from build123d import *

# Parameters (mm, degrees)
F0_W     = 38.4
F0_H     = 28.4
F0_R     = 1.1
F0_R_2   = 4.1
F1_DEPTH = 1.5
F2_W     = 38.4
F2_H     = 1.5
F3_DEPTH = 11
F6_W     = 38.4
F6_H     = 14.2
F7_DEPTH = 25.001
F8_R     = 4.1
F8_R_2   = 1.1
F9_DEPTH = 1.5
F10_R    = 1


with BuildPart() as f1:
    # F0 (on Top) → F1 (new body)
    with BuildSketch(Plane.XY):
        Rectangle(F0_W, F0_H)
        with Locations((-16.2, -7.2)):
            Circle(F0_R, mode=Mode.SUBTRACT)
        with Locations((14.9, -7.2)):
            Circle(F0_R, mode=Mode.SUBTRACT)
        with Locations((-10, 0)):
            Circle(F0_R_2, mode=Mode.SUBTRACT)
        with Locations((-16.2, 7.2)):
            Circle(F0_R, mode=Mode.SUBTRACT)
        with BuildLine():
            ThreePointArc((-3, 4.8), (-1.5355339059, 8.3355339059), (2, 9.8))
            Line((2, 9.8), (11.7, 9.8))
            ThreePointArc((11.7, 9.8), (12.4071067812, 9.5071067812), (12.7, 8.8))
            Line((12.7, 8.8), (12.7, 5.5901699437))
            ThreePointArc((12.7, 5.5901699437), (12.7871290708, 5.1819216533), (13.0333333333, 4.8448139512))
            ThreePointArc((13.0333333333, 4.8448139512), (15.2, 0), (13.0333333333, -4.8448139512))
            ThreePointArc((13.0333333333, -4.8448139512), (12.7871290708, -5.1819216533), (12.7, -5.5901699437))
            Line((12.7, -5.5901699437), (12.7, -8.8))
            ThreePointArc((12.7, -8.8), (12.4071067812, -9.5071067812), (11.7, -9.8))
            Line((11.7, -9.8), (2, -9.8))
            ThreePointArc((2, -9.8), (-1.5355339059, -8.3355339059), (-3, -4.8))
            Line((-3, -4.8), (-3, 4.8))
        make_face(mode=Mode.SUBTRACT)
        with Locations((14.9, 7.2)):
            Circle(F0_R, mode=Mode.SUBTRACT)
    extrude(amount=F1_DEPTH)

    # F2 (on face) → F3 (join)
    with BuildSketch(Plane(origin=(0, 0, 0), x_dir=(1, 0, 0), z_dir=(0, 0, -1))):
        with Locations((0, 13.45)):
            Rectangle(F2_W, F2_H)
    extrude(amount=F3_DEPTH)

    # F5: F1 across plane


with BuildPart() as f1_1:
    add(f1.part)
    add(f1.part.mirror(Plane.XY.offset(-11)))

    # F6 (on face) → F7 (cut, through all)
    with BuildSketch(Plane(origin=(0, 0, -23.5), x_dir=(1, 0, 0), z_dir=(0, 0, -1))):
        with Locations((0, -7.1)):
            Rectangle(F6_W, F6_H)
    extrude(amount=-F7_DEPTH, mode=Mode.SUBTRACT)

    # F8 (on face) → F9 (cut, through all)
    with BuildSketch(Plane.XZ.offset(14.2)):
        with Locations((-10, -11)):
            Circle(F8_R)
        with Locations((-16.2, -3.8)):
            Circle(F8_R_2)
        with Locations((15.4, -3.8)):
            Circle(F8_R_2)
        with BuildLine():
            Line((12.2, -1.2), (2.5, -1.2))
            ThreePointArc((2.5, -1.2), (-1.0355339059, -2.6644660941), (-2.5, -6.2))
            Line((-2.5, -6.2), (-2.5, -15.8))
            ThreePointArc((-2.5, -15.8), (-1.0355339059, -19.3355339059), (2.5, -20.8))
            Line((2.5, -20.8), (12.2, -20.8))
            ThreePointArc((12.2, -20.8), (12.9071067812, -20.5071067812), (13.2, -19.8))
            Line((13.2, -19.8), (13.2, -16.5901699437))
            ThreePointArc((13.2, -16.5901699437), (13.2871290708, -16.1819216533), (13.5333333333, -15.8448139512))
            ThreePointArc((13.5333333333, -15.8448139512), (15.7, -11), (13.5333333333, -6.1551860488))
            ThreePointArc((13.5333333333, -6.1551860488), (13.2871290708, -5.8180783467), (13.2, -5.4098300563))
            Line((13.2, -5.4098300563), (13.2, -2.2))
            ThreePointArc((13.2, -2.2), (12.9071067812, -1.4928932188), (12.2, -1.2))
        make_face()
        with Locations((-16.2, -18.2)):
            Circle(F8_R_2)
        with Locations((15.4, -18.2)):
            Circle(F8_R_2)
    extrude(amount=-F9_DEPTH, mode=Mode.SUBTRACT)

    # F10
    f10_edges = [f1_1.edges().sort_by_distance(p)[0] for p in [
        (-19.2, 0, -22.75),
        (-19.2, 0, 0.75),
        (-5.9, 0, 0.75),
        (-14.1, 0, 0.75),
        (-5.9, 0, -22.75),
        (-14.1, 0, -22.75),
        (-3, 0, -22.75),
        (15.2, 0, -22.75),
        (15.2, 0, 0.75),
        (19.2, 0, -22.75),
        (19.2, 0, 0.75),
        (-3, 0, 0.75),
    ]]
    fillet(f10_edges, radius=F10_R)


solid = f1_1.part
Part model, mm, in its own coordinate system. A direction names the side the tool comes from. Coordinates: 2 decimals unless noted, no trailing zeros. Write each loop counter-clockwise with the first axis right and the second up, starting at its lowest first coordinate (ties: lowest second). Pieces come first, ordered by that corner, then holes. Notation, with made-up numbers: M 67.5,-24 L 81.5,-24 A30 cw 81.5,9 Z; hole C -6,53 d5. An arc over 180 degrees is marked long. Return JSON: item names as keys, results as strings.
1. Saw through at A-A, the plane x = -16.2. Write the cut outline in (y, z).
Determined:
{"outline": "M -14.2,-23.5 L -8.3,-23.5 L -8.3,-22 L -12.7,-22 L -12.7,-19.3 L -14.2,-19.3 Z; M -14.2,-17.1 L -12.7,-17.1 L -12.7,-4.9 L -14.2,-4.9 Z; M -14.2,-2.7 L -12.7,-2.7 L -12.7,0 L -8.3,0 L -8.3,1.5 L -14.2,1.5 Z; M -6.1,-23.5 L 0,-23.5 L 0,-22 L -6.1,-22 Z; M -6.1,0 L 0,0 L 0,1.5 L -6.1,1.5 Z"}
2. Saw through at C-C, the plane x = 3. Write the cut outline in (y, z), then the cut area to 3 significant figures.
Determined:
{"outline": "M -14.2,-23.5 L -9.8,-23.5 L -9.8,-22 L -12.7,-22 L -12.7,-20.8 L -14.2,-20.8 Z; M -14.2,-1.2 L -12.7,-1.2 L -12.7,0 L -9.8,0 L -9.8,1.5 L -14.2,1.5 Z", "area": "16.8 mm²"}
3. Saw through at D-D, the plane z = -11. Write the cut outline in (x, y), then the cut area to 3 significant figures.
Determined:
{"outline": "M -19.2,-14.2 L -14.1,-14.2 L -14.1,-12.7 L -19.2,-12.7 Z; M -5.9,-14.2 L -2.5,-14.2 L -2.5,-12.7 L -5.9,-12.7 Z; M 15.7,-14.2 L 19.2,-14.2 L 19.2,-12.7 L 15.7,-12.7 Z", "area": "18.0 mm²"}
4. Probe L1, parallel to Z at x = -16.2, y = -13.65; L2, parallel to Z at x = 8.5, y = -12.25; L3, parallel to Z at x = -10, y = -13.1. List the from-to ranges inside material, lowest first.
Determined:
{"L1": "-23.5 to -19.3, -17.1 to -4.9, -2.7 to 1.5", "L2": "-23.5 to -22, 0 to 1.5", "L3": "-23.5 to -15.1, -6.9 to 1.5"}
5. Saw through at B-B, the plane y = -11. Write the cut outline in (x, z), then the cut area to 3 significant figures.
Determined:
{"outline": "M -19.2,-23.5 L 19.2,-23.5 L 19.2,-22 L -19.2,-22 Z; M -19.2,0 L 19.2,0 L 19.2,1.5 L -19.2,1.5 Z", "area": "115 mm²"}
6. Flat gauge pins, fed straight in: pin 1 Ø1.2 at (x, z) = (9, 1) entering from +Y; pin 2 Ø9.5 at (x, z) = (-10, -11) entering from +Y; pin 3 Ø3.5 at (x, y) = (-16.2, -7.2) entering from -Z. Where does each tip first touch, or does it go through?
Determined:
{"pin 1": "y = -9.8", "pin 2": "y = -12.7", "pin 3": "z = -23.5"}
7. Pull direction Z, two halves, no side cores. Call faces 4 (the face through (-5, -8, -22)), 5 (the face through (-19.2, -13, -12)), 6 (the face through (-2.5, -13, -11)): pulls with the +Z half, pulls with the -Z half, needs draft (parallel to the pull), parting line crosses it, or undercut.
Determined:
{"face 4": "undercut", "face 5": "needs draft", "face 6": "undercut"}
8. 3-axis set-ups, long thin cutter, end or side, ignore diameter. For faces 1 (the face through (-18.915, -0.301, -22.74)), 2 (the face through (12.915, -13.46, -1.501)), 3 (the face through (-3, -3, -23)): which of +Z, -Z, +X, -X, +Y, -Y reach the whole face in a straight line?
Determined:
{"face 1": "+Z, -Z, -X, +Y", "face 2": "+Y, -Y", "face 3": "+Z, -Z, +Y"}
